The drawing under review shows one solid part. Ordinate dimensions are in mm from its lowest x, y, z. Give positions to 0.01 mm unless a question says otherwise; leave off trailing zeros. Write each loop counter-clockwise with the first axis right and the second up, starting at its lowest first coordinate (ties: lowest second). Pieces come first, ordered by that corner, then holes. Notation, with made-up numbers: (70, 26.5) - (125, 26.5) arc R24 ccw to (125, 50.5) - close; hole circle Ø11 at (9, 32). An arc over 180 degrees is marked (long way). Write each question's results on one line, items separated by ' | '. Start each with the question number.
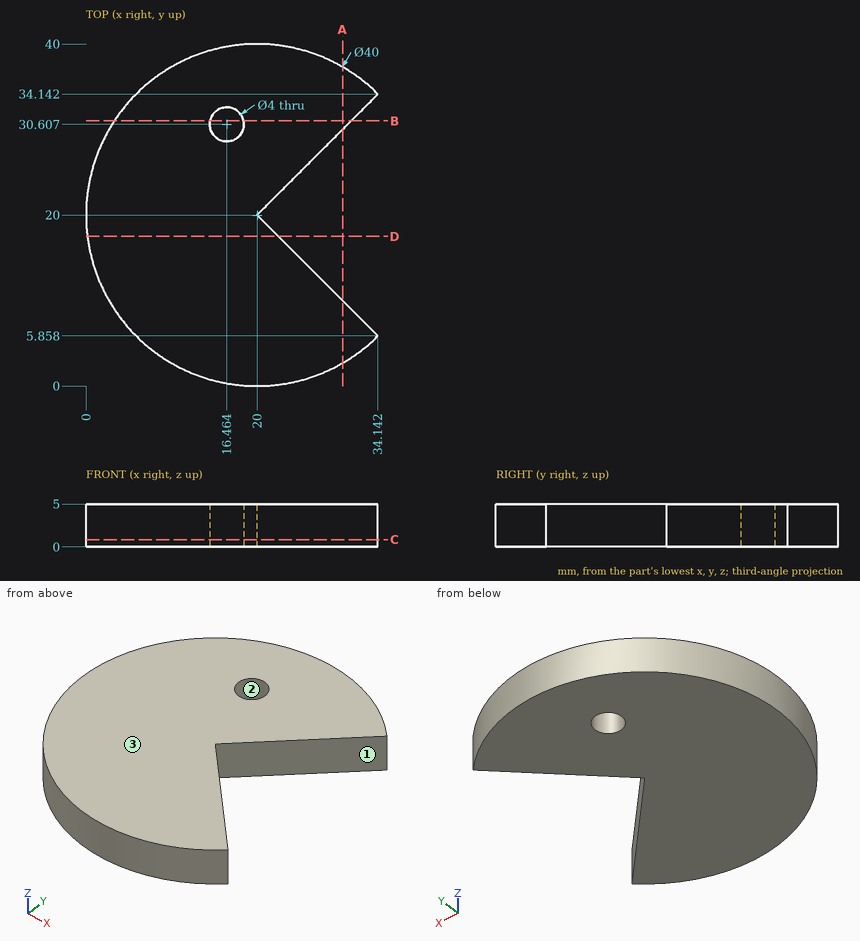
Q1. Add section D-D on y = 17.5. State the section outline as (x, z) points.
Q2. Insertion check: P1, Ø1, axis at y = 6, z = 2.5, coming from the +X side. The pin has a flat end and moves straight along its axis. Give the tip position at first contact, or say it passes through.
Q3. Add section B-B on y = 31. State the section outline as (x, z) points (1 decimal).
Q4. Add section C-C on z = 0.85. State the section outline as (x, y) points (1 decimal), plus the area to 3 significant figures.
Q5. Add section A-A on x = 30. State the section outline as (y, z) points.
Q6. For line 1 along X through (y, z) = (31.5, 4.55) (1 decimal); line 2 along Y through (x, z) = (28, 0.4); line 3 along X through (y, z) = (30.5, 0.3) (1 decimal), list the stretches that pass through material, from the lowest coordinate up. Write a range as [from, to].
Q7. The part is to be moulded in two halves that separate along X. For the marked faces 1, 2 and 3, say which applies: +X half, -X half, draft (parallel to the pull), parting line (faces both ways), or undercut.
Result:
1) outline: (0.16, 0) - (22.5, 0) - (22.5, 5) - (0.16, 5) - close
2) P1: stops at x = 34.14
3) outline: (3.3, 0) - (14.5, 0) - (14.5, 5) - (3.3, 5) - close; (18.4, 0) - (31, 0) - (31, 5) - (18.4, 5) - close
4) outline: (20, 20) - (34.1, 34.1) arc R20 ccw (long way) to (34.1, 5.9) - close; hole circle Ø4 at (16.5, 30.6) | area: 930 mm²
5) outline: (2.68, 0) - (10, 0) - (10, 5) - (2.68, 5) - close; (30, 0) - (37.32, 0) - (37.32, 5) - (30, 5) - close
6) line 1: x = [3.6, 14.7], [18.3, 31.5] | line 2: y = [1.67, 12], [28, 38.33] | line 3: x = [3, 14.5], [18.5, 30.5]
7) face 1: +X half | face 2: undercut | face 3: draft
